Build history of the part. All positions in model axes, mm. A direction names the side the tool comes from. Give positions to 0.01 mm unless a question says otherwise; leave off trailing zeros. Loops run counter-clockwise (first coordinate to the right, second up) from the corner with the lowest first, then second, coordinate; pieces in that order, holes last. Notation, with made-up numbers: (-6, 37) -> (2, 37) arc R31 ccw to (2, 72) -> close; hole circle Ø4 at (45, 28.25). An arc over 180 degrees is marked (long way). Answer as a JSON object with one key per item and string values. Group by question number.
Q1. Band-saw the part on C-C, the plane y = 15. Write the cut outline in (x, z).
Q2. Band-saw the part on B-B, the plane x = -42. Write the cut outline in (y, z), plus the area to 3 significant figures.
Q3. Wall check: probe 1 along Y at (x, z) = (-137.5, 234.5); probe 2 along Y at (x, z) = (243, 354). Give the ranges that are in metal, low to high. Write a range as from..to.
Q4. Band-saw the part on D-D, the plane z = 216.5. Write the cut outline in (x, y).
Q5. Band-saw the part on A-A, the plane z = 107. Write the cut outline in (x, y), plus the area to 3 significant figures.
Q6. Two-plate mould, pull along X, no slides. Class faces 1 (the flat face through (-59, 250, 199)), 2 (the flat face through (230, -3, 266)), 3 (the flat face through (-152.1, -4.2, 677.76)): pulls with the +X half, pulls with the -X half, needs draft (parallel to the pull), parting line crosses it, or undercut.
Q7. Tool access for faces 4 (the flat face through (-54, 230, 211)), 5 (the flat face through (-59, -250, 199)), 6 (the flat face through (90.89, 181.67, 706.5)), 7 (the flat face through (250, -3, 256)): list every direction of +Z, -Z, +X, -X, +Y, -Y with a clear straight run to the whole face (end or side of a thin tool).
Q8. Drop flat-ended pins along their axis: pin 1 (6 mm diameter, centred on y = -175, z = 639.5, fed in from -X); pin 2 (1.5 mm diameter, centred on y = 166.5, z = 647.5, fed in from +X); pin 3 (5 mm diameter, centred on y = -161, z = 570.5, fed in from -X). Give the stop position or say it passes through.
from build123d import *

# Parameters (mm, degrees)
F0_W      = 500
F0_H      = 500
F1_DEPTH  = 20
F2_W      = 500
F2_H      = 500
F2_W_2    = 460
F2_H_2    = 460
F3_DEPTH  = 500
F4_R      = 77.3069770254
F5_DEPTH  = 500.001
F6_W      = 600
F6_H      = 600
F7_DEPTH  = 20
F8_DEPTH  = 300
F10_DEPTH = 600.001
F12_DEPTH = 25


with BuildPart() as f1:
    # F0 (on Top) → F1 (new body)
    with BuildSketch(Plane.XY):
        Rectangle(F0_W, F0_H)
    extrude(amount=F1_DEPTH)

    # F2 (on face) → F3 (join)
    with BuildSketch(Plane.XY.offset(20)):
        Rectangle(F2_W, F2_H)
        Rectangle(F2_W_2, F2_H_2, mode=Mode.SUBTRACT)
    extrude(amount=F3_DEPTH)

    # F4 (on face) → F5 (cut, through all)
    with BuildSketch(Plane.XZ.offset(250)):
        with Locations((0, 267.239511013)):
            Circle(F4_R)
    extrude(amount=-F5_DEPTH, mode=Mode.SUBTRACT)

    # F6 (on face) → F7 (join)
    with BuildSketch(Plane.XY.offset(520)):
        Rectangle(F6_W, F6_H)
    extrude(amount=F7_DEPTH)

    # F8 (add): a face of the model
    f8_faces = [f1.faces().sort_by_distance(p)[0] for p in [
        (0, 0, 540),
    ]]
    extrude(f8_faces, amount=F8_DEPTH)

    # F9 (on face) → F10 (cut, through all)
    with BuildSketch(Plane.XZ.offset(300)):
        Polygon((-300, 520), (0, 840), (-300, 840), align=None)
        Polygon((300, 840), (0, 840), (300, 520), align=None)
    extrude(amount=-F10_DEPTH, mode=Mode.SUBTRACT)

    # F11 (on face) → F12 (cut)
    with BuildSketch(Plane(origin=(419.1268191268, 0, 392.9313929314), x_dir=(0, 1, 0), z_dir=(0.7295372041, 0, 0.6839411289))):
        Polygon((-300, 174.1770074884), (0, 612.8112514777), (-300, 612.8112514777), align=None)
        Polygon((300, 612.8112514777), (0, 612.8112514777), (300, 174.1770074884), align=None)
    extrude(amount=-F12_DEPTH, mode=Mode.SUBTRACT)


solid = f1.part
Worked answers:
{
 "1": {"outline": "(-300, 520) -> (-250, 520) -> (-250, 0) -> (250, 0) -> (250, 520) -> (300, 520) -> (15, 824) -> (-3.24, 806.9) -> (-17.13, 821.72) -> close; hole (-230, 20) -> (230, 20) -> (230, 520) -> (-230, 520) -> close"},
 "2": {"outline": "(-300, 520) -> (-250, 520) -> (-250, 332.14) -> (-230, 332.14) -> (-230, 520) -> (230, 520) -> (230, 332.14) -> (250, 332.14) -> (250, 520) -> (300, 520) -> (300, 795.2) -> (-300, 795.2) -> close; (-250, 0) -> (250, 0) -> (250, 202.34) -> (230, 202.34) -> (230, 20) -> (-230, 20) -> (-230, 202.34) -> (-250, 202.34) -> close", "area": "190,000 mm2"},
 "3": {"probe 1": "-250..-230, 230..250", "probe 2": "-250..250"},
 "4": {"outline": "(-250, -250) -> (-58.33, -250) -> (-58.33, -230) -> (-230, -230) -> (-230, 230) -> (-58.33, 230) -> (-58.33, 250) -> (-250, 250) -> close; (58.33, -250) -> (250, -250) -> (250, 250) -> (58.33, 250) -> (58.33, 230) -> (230, 230) -> (230, -230) -> (58.33, -230) -> close"},
 "5": {"outline": "(-250, -250) -> (250, -250) -> (250, 250) -> (-250, 250) -> close; hole (-230, -230) -> (230, -230) -> (230, 230) -> (-230, 230) -> close", "area": "38,400 mm2"},
 "6": {"face 1": "needs draft", "face 2": "undercut", "face 3": "pulls with the -X half"},
 "7": {"face 4": "none", "face 5": "-Z, +X, -X, -Y", "face 6": "+Z, +Y", "face 7": "-Z, +X, +Y, -Y"},
 "8": {"pin 1": "x = -190.78", "pin 2": "x = 181.17", "pin 3": "x = -255"}
}
